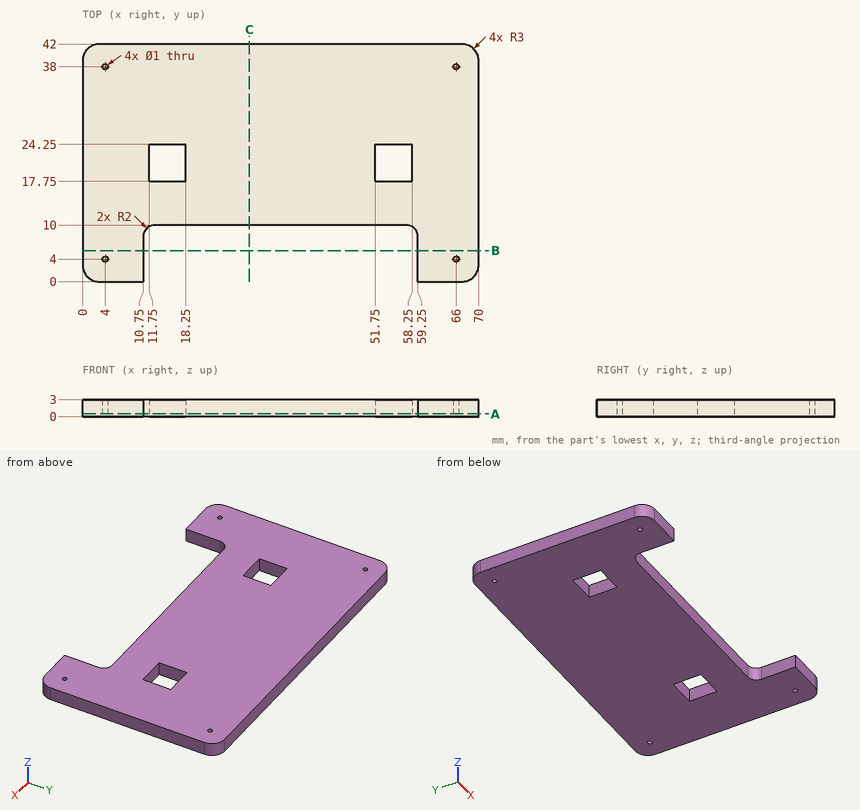
Geometry check sheet. Reference: drawing and pictorial views, mm from the part's lowest x, y, z. Give positions to 0.01 mm unless a question says otherwise; leave off trailing zeros. Write each loop counter-clockwise with the first axis right and the second up, starting at its lowest first coordinate (ties: lowest second). Pieces come first, ordered by that corner, then holes. Notation, with made-up numbers: M 55.5,6 L 94.5,6 A21 cw 94.5,37 Z; hole C 69,49 d2. An arc over 180 degrees is marked long. Put each result on its own line as item: value. Start each with the question number.
1. Section check C-C (x = 29.5). Record the cut outline in (y, z).
2. Go/stop test with a flat-tipped pin: pin 1 Ø0.9 at (x, z) = (46, 1.5) entering from -Y. Record where the tip stops, or that it passes through.
3. Scan lines: line 1 along Y through (x, z) = (4, 1.2); line 2 along X through (y, z) = (38, 0.8); line 3 along X through (y, z) = (22, 2.6). Record each from-to range of solid material in increasing order. Write a range as [from, to].
4. Section check B-B (y = 5.5). Record the cut outline in (x, z), and give its area (3 significant figures).
5. Section check A-A (z = 0.5). Record the cut outline in (x, y), and give its area (3 significant figures).
Answer list:
1. outline: M 10,0 L 42,0 L 42,3 L 10,3 Z
2. pin 1: y = 10
3. line 1: [0, 3.5], [4.5, 37.5], [38.5, 42]
3. line 2: [0, 3.5], [4.5, 65.5], [66.5, 70]
3. line 3: [0, 11.75], [18.25, 51.75], [58.25, 70]
4. outline: M 0,0 L 10.75,0 L 10.75,3 L 0,3 Z; M 59.25,0 L 70,0 L 70,3 L 59.25,3 Z
4. area: 64.5 mm2
5. outline: M 0,3 A3 ccw 3,0 L 10.75,0 L 10.75,8 A2 cw 12.75,10 L 57.25,10 A2 cw 59.25,8 L 59.25,0 L 67,0 A3 ccw 70,3 L 70,39 A3 ccw 67,42 L 3,42 A3 ccw 0,39 Z; hole C 4,4 d1; hole C 4,38 d1; hole M 11.75,17.75 L 18.25,17.75 L 18.25,24.25 L 11.75,24.25 Z; hole M 51.75,17.75 L 58.25,17.75 L 58.25,24.25 L 51.75,24.25 Z; hole C 66,4 d1; hole C 66,38 d1
5. area: 2,360 mm2
